Autodesk Fusion 360 part; units mm, degrees
sketch "Sketch1" plane through (0, 0, 0) normal (0, 0, 1) x (1, 0, 0)
  line L0 (10, 0) -> (210, 0)
  line L1 (220, 10) -> (220, 210)
  line L2 (210, 220) -> (10, 220)
  line L3 (0, 210) -> (0, 10)
  line L4 (83, 0) -> (138, 0)
  line L5 (138, 0) -> (138, 55)
  line L6 (128, 65) -> (93, 65)
  line L7 (83, 55) -> (83, 0)
  line L8 (52.5, 220) -> (127.5, 220)
  line L9 (127.5, 220) -> (127.5, 165)
  line L10 (117.5, 155) -> (62.5, 155)
  line L11 (52.5, 165) -> (52.5, 220)
  line L12 (52.5, 165) -> (62.5, 155)
  line L13 (117.5, 155) -> (127.5, 165)
  line L14 (83, 55) -> (93, 65)
  line L15 (128, 65) -> (138, 55)
  line L16 (0, 25) -> (10, 25)
  line L17 (10, 25) -> (10, 95)
  line L18 (10, 95) -> (0, 95)
  line L19 (0, 95) -> (0, 25)
  line L20 (0, 125) -> (10, 125)
  line L21 (10, 125) -> (10, 195)
  line L22 (10, 195) -> (0, 195)
  line L23 (0, 195) -> (0, 125)
  line L24 (10, 220) -> (0, 210)
  line L25 (210, 220) -> (220, 210)
  line L26 (0, 10) -> (10, 0)
  line L27 (210, 0) -> (220, 10)
  line L28 (0, 95) -> (10, 85)
  line L29 (0, 125) -> (10, 135)
  line L30 (0, 195) -> (10, 185)
  line L31 (0, 25) -> (10, 35)
  line L32 (110, 0) -> (110, 220) construction
  line L33 (210, 195) -> (220, 195)
  line L34 (220, 195) -> (210, 185)
  line L35 (210, 125) -> (210, 195)
  line L36 (220, 125) -> (210, 135)
  line L37 (220, 125) -> (210, 125)
  line L38 (210, 95) -> (220, 95)
  line L39 (210, 25) -> (210, 95)
  line L40 (220, 95) -> (210, 85)
  line L41 (220, 25) -> (210, 25)
  line L42 (220, 25) -> (210, 35)
  line L43 (0, 110) -> (220, 110) construction
  line L44 (150, 142) -> (70, 142) construction
  line L45 (70, 142) -> (70, 78) construction
  line L46 (70, 78) -> (150, 78) construction
  line L47 (150, 78) -> (150, 142) construction
  line L48 (150, 142) -> (70, 78) construction
  line L49 (70, 142) -> (150, 78) construction
  line L50 (102, 65) -> (102, 73)
  line L51 (102, 73) -> (113, 73)
  line L52 (113, 73) -> (113, 70)
  line L53 (113, 70) -> (105, 70)
  line L54 (105, 70) -> (105, 65)
  line L55 (102, 155) -> (102, 147)
  line L56 (102, 147) -> (113, 147)
  line L57 (113, 150) -> (105, 150)
  line L58 (113, 147) -> (113, 150)
  line L59 (105, 150) -> (105, 155)
  line L60 (42.5, 220) -> (52.5, 210)
  line L61 (127.5, 210) -> (137.5, 220)
  line L62 (138, 10) -> (148, 0)
  line L63 (83, 10) -> (73, 0)
  point P0 (220, 0)
  point P1 (0, 220)
  point P2 (52.5, 155)
  point P3 (127.5, 155)
  point P4 (83, 65)
  point P5 (138, 65)
  point P6 (220, 220)
  point P7 (110, 110)
  point P8 (110, 110)
  dimension "d1" = 220
  dimension "d2" = 220
  dimension "d3" = 83
  dimension "d4" = 138
  dimension "d5" = 65
  dimension "d6" = 52.5
  dimension "d7" = 127.5
  dimension "d8" = 65
  dimension "d9" = 10
  dimension "d10" = 10
  dimension "d11" = 10
  dimension "d12" = 10
  dimension "d13" = 10
  dimension "d14" = 10
  dimension "d15" = 10
  dimension "d16" = 10
  dimension "d17" = 95
  dimension "d18" = 25
  dimension "d19" = 10
  dimension "d20" = 195
  dimension "d21" = 125
  dimension "d22" = 10
  dimension "d23" = 10
  dimension "d24" = 10
  dimension "d25" = 10
  dimension "d26" = 10
  dimension "d27" = 10
  dimension "d28" = 10
  dimension "d29" = 10
  dimension "d30" = 10
  dimension "d31" = 80
  dimension "d32" = 64
  dimension "d41" = 102
  dimension "d42" = 3
  dimension "d44" = 3
  dimension "d45" = 11
  dimension "d46" = 8
  dimension "d60" = 10
  dimension "d61" = 10
  dimension "d62" = 10
  dimension "d63" = 10
extrude "Extrude1" add sketch "Sketch1" along normal blind 4 contours L0 L1 L2 L3 L5 L6 L7 L9 L10 L11 L12 L13 L14 L15 L16 L17 L18 L20 L21 L22 L24 L25 L26 L27 L33 L35 L37 L38 L39 L41 L50 L51 L52 L53 L54 L55 L56 L57 L58 L59 L60 L61 L62 L63 | L16 L17 L31 | L17 L18 L28 | L20 L21 L29 | L21 L22 L30 | L39 L41 L42 | L38 L39 L40 | L35 L36 L37 | L33 L34 L35
hole "Hole1" at (70, 142, 0) at (70, 78, 0) direction (0, 0, 1) diameter 5 end through all
hole "Hole2" at (150, 78, 0) at (150, 142, 0) direction (0, 0, 1) diameter 7.2 depth 4 tip angle 118
sketch "Sketch2" plane through (0, 0, 4) normal (0, 0, 1) x (-1, 0, 0)
  circle A0 centre (-150, -78) radius 3.6
  circle A1 centre (-150, -142) radius 3.6
  circle A2 centre (-70, -142) radius 2.5
  circle A3 centre (-70, -78) radius 2.5
  line L0 (-102, -155) -> (-62.5, -155)
  line L1 (-62.5, -155) -> (-52.5, -165)
  line L2 (-52.5, -165) -> (-52.5, -210)
  line L3 (-42.5, -220) -> (-10, -220)
  line L4 (-10, -220) -> (0, -210)
  line L5 (0, -210) -> (0, -195)
  line L6 (0, -195) -> (-10, -185)
  line L7 (-10, -185) -> (-10, -135)
  line L8 (-10, -135) -> (0, -125)
  line L9 (0, -125) -> (0, -95)
  line L10 (0, -95) -> (-10, -85)
  line L11 (-10, -85) -> (-10, -35)
  line L12 (-10, -35) -> (0, -25)
  line L13 (0, -25) -> (0, -10)
  line L14 (0, -10) -> (-10, 0)
  line L15 (-10, 0) -> (-73, 0)
  line L16 (-83, -10) -> (-83, -55)
  line L17 (-83, -55) -> (-93, -65)
  line L18 (-93, -65) -> (-102, -65)
  line L19 (-102, -65) -> (-102, -73)
  line L20 (-102, -73) -> (-113, -73)
  line L21 (-113, -73) -> (-113, -70)
  line L22 (-113, -70) -> (-105, -70)
  line L23 (-105, -70) -> (-105, -65)
  line L24 (-105, -65) -> (-128, -65)
  line L25 (-128, -65) -> (-138, -55)
  line L26 (-138, -55) -> (-138, -10)
  line L27 (-148, 0) -> (-210, 0)
  line L28 (-210, 0) -> (-220, -10)
  line L29 (-220, -10) -> (-220, -25)
  line L30 (-220, -25) -> (-210, -35)
  line L31 (-210, -35) -> (-210, -85)
  line L32 (-210, -85) -> (-220, -95)
  line L33 (-220, -95) -> (-220, -125)
  line L34 (-220, -125) -> (-210, -135)
  line L35 (-210, -135) -> (-210, -185)
  line L36 (-210, -185) -> (-220, -195)
  line L37 (-220, -195) -> (-220, -210)
  line L38 (-220, -210) -> (-210, -220)
  line L39 (-210, -220) -> (-137.5, -220)
  line L40 (-127.5, -210) -> (-127.5, -165)
  line L41 (-127.5, -165) -> (-117.5, -155)
  line L42 (-117.5, -155) -> (-105, -155)
  line L43 (-105, -155) -> (-105, -150)
  line L44 (-105, -150) -> (-113, -150)
  line L45 (-113, -150) -> (-113, -147)
  line L46 (-113, -147) -> (-102, -147)
  line L47 (-102, -147) -> (-102, -155)
  line L48 (0, -110) -> (-220, -110) construction
  line L49 (-10, 0) -> (-210, 0) construction
  line L50 (0, -10) -> (-220, -10) construction
  line L51 (0, -210) -> (-220, -210) construction
  line L52 (-138, -10) -> (-148, 0)
  line L53 (-137.5, -220) -> (-127.5, -210)
  line L54 (-52.5, -210) -> (-42.5, -220)
  line L55 (-73, 0) -> (-83, -10)
  point P0 (-15, -110)
  point P1 (-80, -110)
  point P2 (-140, -110)
  point P3 (-210, -110)
  point P4 (-15, -210)
  point P5 (-136, -210)
  point P6 (-206, -210)
  point P7 (-15, -10)
  point P8 (-70, -10)
  point P9 (-150, -10)
  point P10 (-205, -10)
  point P11 (-148, -164)
  dimension "d47" = 110
  dimension "d48" = 10
  dimension "d49" = 15
  dimension "d50" = 80
  dimension "d51" = 140
  dimension "d52" = 210
  dimension "d53" = 15
  dimension "d54" = 136
  dimension "d55" = 206
  dimension "d56" = 15
  dimension "d57" = 70
  dimension "d58" = 150
  dimension "d59" = 205
  dimension "d70" = 148
  dimension "d71" = 164
hole "Hole3" at (15, 210, 4) at (136, 210, 4) at (206, 210, 4) at (210, 110, 4) at (140, 110, 4) at (80, 110, 4) at (15, 110, 4) at (15, 10, 4) at (70, 10, 4) at (150, 10, 4) at (205, 10, 4) direction (0, 0, -1) diameter 3.332 depth 4 tip angle 118
hole "Hole5" at (148, 164, 4) direction (0, 0, -1) diameter 3.332 depth 4 tip angle 118
ref_plane "WorkPlane1" through (110, 110, 2) normal (-1, 0, 0) x (0, -1, 0)
equation "d10 = d9"
equation "d12 = d11"
equation "d14 = d13"
equation "d16 = d15"
equation "d24 = d23"
equation "d26 = d25"
equation "d28 = d27"
equation "d30 = d29"
Geometry: final body of the model. Coordinates: model frame, mm. A direction names the side the tool comes from. Round coordinates to 2 decimals unless told otherwise and drop trailing zeros. Loops run counter-clockwise (first coordinate to the right, second up) from the corner with the lowest first, then second, coordinate; pieces in that order, holes last.
Q1. Section A-A on y = 142. Return loops of the section in (x, z).
Q2. Material intervals for L1, parallel to X at y = 210, z = 1.7; L2, parallel to X at y = 10, z = 3; L3, parallel to Y at x = 150, z = 1.5, sorted ascending.
Q3. Pull-direction query (X, two-part tool) for faces 5 (the flat face through (5, 30, 2)), 6 (the flat face through (108, 112, 0)), 7 (the flat face through (78, 5, 2)), 8 (the flat face through (88, 60, 2)); classes: released by +X, released by -X, zero draft, split by the parting line, or undercut.
Q4. Section D-D on y = 58.5. Return loops of the section in (x, z).
Q5. Access query for faces 1 (the flat face through (215, 190, 2)), 2 (the flat face through (122.4, 159.9, 2)), 3 (the cylindrical face through (147.567, 139.347, 2.028)), 4 (the flat face through (5, 90, 2)). Directions: +Z, -Z, +X, -X, +Y, -Y. A direction counts if a zero-diameter tool reaches every point of the face in a straight line with its end or side. Return the directions, or none.
Q6. Section C-C on z = 2.95. State how many separate pieces and enclosed holes the cut face has, plus the area to 3 significant figures.
Q7. Pin query (flat end, axial travel): P1, Ø2, axis at x = 120, z = 2.5, coming from the -Y side; P2, Ø1, axis at y = 29.5, z = 2, coming from the -X side. Return the tip coordinate at first contact, or that it passes through.
Q8. Section B-B on y = 171. Return loops of the section in (x, z).
Evaluation:
1. outline: (10, 0) - (67.5, 0) - (67.5, 4) - (10, 4) - close; (72.5, 0) - (146.4, 0) - (146.4, 4) - (72.5, 4) - close; (153.6, 0) - (210, 0) - (210, 4) - (153.6, 4) - close
2. L1: x = 0 to 13.33, 16.67 to 52.5, 127.5 to 134.33, 137.67 to 204.33, 207.67 to 220
2. L2: x = 0 to 13.33, 16.67 to 68.33, 71.67 to 83, 138 to 148.33, 151.67 to 203.33, 206.67 to 220
2. L3: y = 0 to 8.33, 11.67 to 74.4, 81.6 to 138.4, 145.6 to 220
3. face 5: released by -X
3. face 6: zero draft
3. face 7: undercut
3. face 8: undercut
4. outline: (10, 0) - (86.5, 0) - (86.5, 4) - (10, 4) - close; (134.5, 0) - (210, 0) - (210, 4) - (134.5, 4) - close
5. face 1: +Z, -Z, +X
5. face 2: +Z, -Z, +Y
5. face 3: +Z, -Z
5. face 4: +Z, -Z, -X
6. separate pieces: 1
6. enclosed holes: 16
6. area: 37,000 mm2
7. P1: stops at y = 65
7. P2: stops at x = 4
8. outline: (10, 0) - (52.5, 0) - (52.5, 4) - (10, 4) - close; (127.5, 0) - (210, 0) - (210, 4) - (127.5, 4) - close
